from build123d import *

# Parameters (mm, degrees)
SKETCH2_OUTSIDE_W  = 78.56
SKETCH2_OUTSIDE_H  = 78.56
CUT_EXTRUDE1_DEPTH = 10.525
FILLET1_R          = 0.381


with BuildPart() as part:
    # Sketch1 → Revolve1 (revolve)
    with BuildSketch(Plane(origin=(0, 0, 0), x_dir=(0, 0, -1), z_dir=(1, 0, 0)), mode=Mode.PRIVATE) as revolve1_sk:
        with BuildLine():
            Line((0, 29.614428494), (0, 6.477))
            Line((0, 6.477), (-3.175, 6.477))
            Line((-3.175, 6.477), (-4.5212, 7.8232))
            Line((-4.5212, 7.8232), (-11.3538, 7.8232))
            Line((-11.3538, 7.8232), (-12.7, 6.477))
            Line((-12.7, 6.477), (-12.7, 0))
            Line((-12.7, 0), (9.525, 0))
            ThreePointArc((9.525, 0), (7.085159222, 15.554259867), (0, 29.614428494))
        make_face()
    revolve(revolve1_sk.sketch.rotate(Axis((0, 0, 0), (0, 0, 1)), 90), axis=Axis((0, 0, 0), (0, 0, 1)))  # turned: the seam where the file's is

    # Sketch2 outside → Cut-Extrude1 (cut, through all)
    with BuildSketch(Plane.XY):
        Rectangle(SKETCH2_OUTSIDE_W, SKETCH2_OUTSIDE_H)
        Polygon((0, 14.664696837), (-12.7, 7.332348419), (-12.7, -7.332348419), (0, -14.664696837), (12.7, -7.332348419), (12.7, 7.332348419), align=None, mode=Mode.SUBTRACT)
    extrude(amount=-CUT_EXTRUDE1_DEPTH, mode=Mode.SUBTRACT)

    # Fillet1
    fillet1_edges = [part.edges().sort_by_distance(p)[0] for p in [
        (6.477, 0, 0),
    ]]
    fillet(fillet1_edges, radius=FILLET1_R)


solid = part.part
Model file for the job. Use its own axes, mm. A direction names the side the tool comes from. Round coordinates to 2 decimals unless told otherwise and drop trailing zeros. Loops run counter-clockwise (first coordinate to the right, second up) from the corner with the lowest first, then second, coordinate; pieces in that order, holes last. Notation, with made-up numbers: (-27.5, 53) - (-2.5, 53) arc R18 cw to (-2.5, 70) - close; hole circle Ø7 at (-21, -5). An arc over 180 degrees is marked (long way). Write each question's results on one line, items separated by ' | '.
(1) Saw through at B-B, the plane z = -2.75. List the corners of the cut face in (x, y).
Answer below:
outline: (-12.7, -7.33) - (0, -14.66) - (12.7, -7.33) - (12.7, 7.33) - (0, 14.66) - (-12.7, 7.33) - close
(2) Saw through at C-C, the plane z = 0.75. List the corners of the cut face in (x, y), then the cut area to 3 significant figures.
Answer below:
outline: circle Ø12.95 at (0, 0) | area: 132 mm^2
(3) Saw through at A-A, the plane y = 0. List the corners of the cut face in (x, z) (3 decimals), then the cut area to 3 significant figures.
Answer below:
outline: (-12.7, -7.912) arc R50.8 ccw to (12.7, -7.912) - (12.7, 0) - (6.858, 0) arc R0.381 cw to (6.477, 0.381) - (6.477, 3.175) - (7.823, 4.521) - (7.823, 11.354) - (6.477, 12.7) - (-6.477, 12.7) - (-7.823, 11.354) - (-7.823, 4.521) - (-6.477, 3.175) - (-6.477, 0.381) arc R0.381 cw to (-6.858, 0) - (-12.7, 0) - close | area: 415 mm^2
(4) 3-axis set-ups, long thin cutter, end or side, ignore diameter. For faces 1 (the cylindrical face through (-7.46, -2.35, 7.99)), 2 (the flat face through (6.26, -11.05, -3.9)): which of +Z, -Z, +X, -X, +Y, -Y reach the whole face in a straight line?
Answer below:
face 1: +Z | face 2: +Z, -Z, +X, -Y
(5) Mould opens along Z. For faces 3 (the cylindrical face through (1.404, 6.323, 1.798)), 4 (the flat face through (0, 0, 12.7)), 5 (the flat face through (-6.26, 11.05, -3.9)) say: released by +Z, released by -Z, zero draft, split by the parting line, or undercut.
Answer below:
face 3: undercut | face 4: released by +Z | face 5: zero draft
(6) Wall check: L1, parallel to Y at x = -0.25, z = 8.75; L2, parallel to Z at x = 11, y = -5; L3, parallel to Z at x = -5.5, y = 2.25. Give the ranges that are in metal, low to high.
Answer below:
L1: y = -7.82 to 7.82 | L2: z = -8.07 to 0 | L3: z = -9.18 to 12.7
(7) Pin check, flat tips, straight feed: pin 1 (3 mm diameter, centred on y = 11, z = -4.5, fed in from -X); pin 2 (2 mm diameter, centred on x = 0.5, z = -6, fed in from +Y); pin 3 (8 mm diameter, centred on x = 4.5, z = -0.5, fed in from +Y). Stop position of each tip, or through.
Answer below:
pin 1: stops at x = -8.95 | pin 2: stops at y = 14.66 | pin 3: stops at y = 14.38
